from build123d import *

# Parameters (mm, degrees)
CYLINDER011_R     = 5
CYLINDER011_DEPTH = 15
PAD_DEPTH         = 5
ARRAY006_COUNT    = 4


with BuildPart() as cylinder011:
    # Cylinder011 → Cylinder011 (new body)
    with BuildSketch(Plane.XY):
        Circle(CYLINDER011_R)
    extrude(amount=CYLINDER011_DEPTH)


with BuildPart() as sphere:
    # Sphere → Sphere (revolve)
    with BuildSketch(Plane(origin=(0, 0, 17), x_dir=(1, 0, 0), z_dir=(0, -1, 0))):
        with BuildLine():
            ThreePointArc((0, -6.5), (6.5, 0), (0, 6.5))
            Line((0, 6.5), (0, -6.5))
        make_face()
    revolve(axis=Axis((0, 0, 17), (0, 0, 1)))


with BuildPart() as obj1:
    # Sketch → Pad (new body)
    with BuildSketch(Plane.XY):
        Polygon((0, 7.5), (17.5, 7.5), (25, 0), (17.5, -7.5), (0, -7.5), align=None)
    extrude(amount=PAD_DEPTH)

    # Array006: obj1 ×4 about axis
    array006_axis = Axis((0, 0, 0), (0, 0, 1))


with BuildPart() as obj1_1:
    add(obj1.part)
    for i in range(1, ARRAY006_COUNT):
        add(obj1.part.rotate(array006_axis, i * 360 / ARRAY006_COUNT))

    # Fusion017: union Cylinder011, Sphere
    add(cylinder011.part)
    add(sphere.part)


solid = obj1_1.part
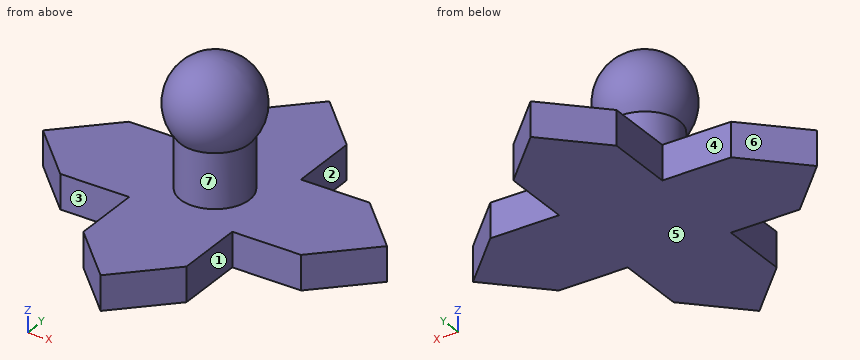
Input: part model. Units: mm. Frame: model coordinates. Face numbers are marked on the shaded views. A direction names the side the tool comes from. Round coordinates to 2 decimals unless told otherwise and drop trailing zeros. Order: outer loops, then holes, each group sorted by start corner. A loop starts at its lowest first (then second) coordinate and runs counter-clockwise, first axis right, second up.
1. Mould query, pull axis Z, two halves, no side actions, for the marked faces 5, 6 and 7. Classes: released by +Z, released by -Z, zero draft, split by the parting line, or undercut.
The answers:
face 5: released by -Z
face 6: zero draft
face 7: undercut
2. Material intervals for line 1 (Z direction, x = -1, y = -12.5); line 2 (Y direction, x = -15, z = 1); line 3 (X direction, y = -4, z = 15.25), sorted ascending.
The answers:
line 1: z = 0 to 5
line 2: y = -7.5 to 7.5
line 3: x = -4.82 to 4.82
3. Pin query (flat end, axial travel): P1, Ø1.5, axis at x = -14, z = 3.5, coming from the +Y side; P2, Ø1, axis at x = -5, z = 13, coming from the +Y side; P3, Ø2.5, axis at y = 12.5, z = 3, coming from the -X side; P4, Ø5, axis at y = -8.5, z = 8.5, coming from the -X side. Return the tip coordinate at first contact, or that it passes through.
The answers:
P1: stops at y = 7.5
P2: stops at y = 2.72
P3: stops at x = -7.5
P4: passes through
4. Cut plane B-B, the plane y = -18.5. Output: boundary loops of the cut face in (x, z), then the cut area to 3 significant figures.
The answers:
outline: (-6.5, 0) - (6.5, 0) - (6.5, 5) - (-6.5, 5) - close
area: 65.0 mm2
5. Cut plane D-D, the plane y = 9. Output: boundary loops of the cut face in (x, z).
The answers:
outline: (-7.5, 0) - (7.5, 0) - (7.5, 5) - (-7.5, 5) - close
6. Set-up query: the marked faces 1, 2, 3 and 4. Return all of +Z, -Z, +X, -X, +Y, -Y with unobstructed straight access to the full face (end or side cutting, diameter ignored); none if empty.
The answers:
face 1: +Z, -Z, +X, -Y
face 2: +Z, -Z, +X, +Y
face 3: +Z, -Z, -X, -Y
face 4: +Z, -Z, -X, +Y
7. Cut plane C-C, the plane z = 7.25. Output: boundary loops of the cut face in (x, y).
The answers:
outline: circle Ø10 at (0, 0)
8. Cut plane A-A, the plane x = -4. Output: boundary loops of the cut face in (y, z).
The answers:
outline: (-21, 0) - (21, 0) - (21, 5) - (3, 5) - (3, 12.85) arc R5.12 ccw (long way) to (-3, 12.85) - (-3, 5) - (-21, 5) - close
